Part print with two shaded views. Sizes in mm from the minimum x, y, z corner. A direction names the side the tool comes from. Round coordinates to 2 decimals unless told otherwise and drop trailing zeros. Write each loop counter-clockwise with the first axis right and the second up, starting at its lowest first coordinate (ties: lowest second). Pieces come first, ordered by that corner, then holes. Notation, with made-up numbers: (58.25, 27) -> (84.25, 27) arc R16 ccw to (84.25, 34) -> close; hole circle Ø8 at (4.25, -36). An arc over 180 degrees is marked (long way). Return JSON: item names as keys, results as strings. Group by question number.
(1) Saw through at A-A (x = 17.25). List the corners of the cut face in (y, z).
(2) Saw through at C-C (x = 40.5). List the corners of the cut face in (y, z), plus the area to 3 significant figures.
(3) Mould opens along X. For the marked faces 6, 7, 8 and 9 say: +X half, -X half, draft (parallel to the pull), parting line (faces both ways), or undercut.
(4) Drill centre lines: L1, parallel to X at y = 20.1, z = 8 (3 decimals); L2, parallel to X at y = 21.2, z = 8 (3 decimals); L3, parallel to Z at x = 17.25, y = 4. Where is each one in solid material? Low to high. Write a range as from..to.
(5) Tool access for the marked faces 1, 2, 3, 4 and 5: list every direction of +Z, -Z, +X, -X, +Y, -Y with a clear straight run to the whole face (end or side of a thin tool).
(6) Drop flat-ended pins along their axis: pin 1 Ø3 at (x, z) = (53.25, 3.5) entering from +Y; pin 2 Ø6.5 at (x, z) = (41, 8.5) entering from -Y; pin 3 Ø1.8 at (y, z) = (13.5, 11.5) entering from -X; pin 4 Ø1.5 at (x, z) = (47, 14) entering from +Y. Give the stop position or say it passes through.
(7) Saw through at B-B (z = 3.5). State how many separate pieces and enclosed holes the cut face has, plus the area to 3 significant figures.
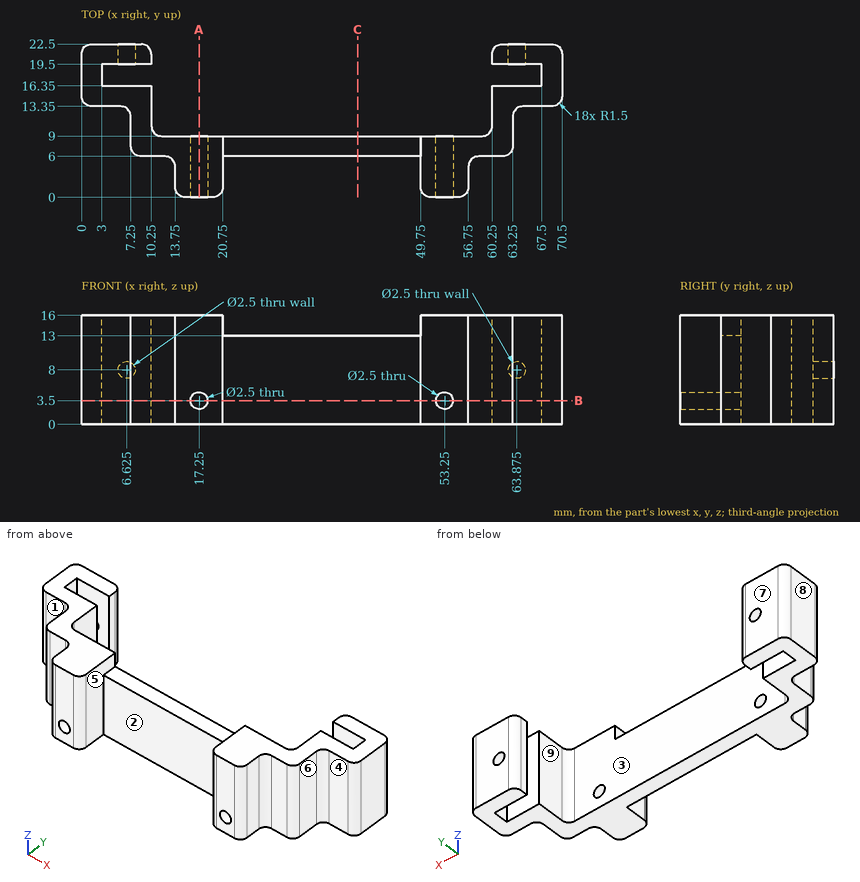
Computed values:
{
 "1": {"outline": "(0, 0) -> (9, 0) -> (9, 2.25) -> (0, 2.25) -> close; (0, 4.75) -> (9, 4.75) -> (9, 16) -> (0, 16) -> close"},
 "2": {"outline": "(6, 0) -> (9, 0) -> (9, 13) -> (6, 13) -> close", "area": "39.0 mm2"},
 "3": {"face 6": "+X half", "face 7": "draft", "face 8": "-X half", "face 9": "undercut"},
 "4": {"L1": "0..5.375, 7.875..10.25, 60.25..62.625, 65.125..70.5", "L2": "0.013..5.375, 7.875..10.237, 60.263..62.625, 65.125..70.487", "L3": "0..2.25, 4.75..16"},
 "5": {"face 1": "+Z, -Z, -X, -Y", "face 2": "+Z, -Z, -Y", "face 3": "+Z, -Z, +Y", "face 4": "+Z, -Z, +X, -Y", "face 5": "+Z, -Y"},
 "6": {"pin 1": "y = 9", "pin 2": "y = 6", "pin 3": "x = 0.07", "pin 4": "through"},
 "7": {"separate pieces": "3", "enclosed holes": "0", "area": "372 mm2"}
}
